Job drawing, mm, ordinate dimensions from the low corner. One solid piece. Coordinates: 2 decimals unless noted, no trailing zeros. Loops run counter-clockwise (first coordinate to the right, second up) from the corner with the lowest first, then second, coordinate; pieces in that order, holes last. Notation, with made-up numbers: (31.5, 59.5) - (39.5, 59.5) arc R26 cw to (39.5, 73.5) - close; hole circle Ø6 at (56, 80.5). An arc over 180 degrees is marked (long way). Use a Markdown table: item, result. Add a question column.
1) Band-saw the part on B-B (x = 5). Give the number of separate pieces and of enclosed holes in the cut face, plus the area to 3 significant figures.
2) Drop flat-ended pins along their axis: P1, Ø6, axis at y = 24, z = 5, coming from the +X side; P2, Ø1, axis at y = 23, z = 7, coming from the -X side; P3, Ø0.8, axis at x = 5, z = 18, coming from the -Y side; P4, Ø7, axis at x = 5, y = 7, coming from the +Z side. Give the stop position or say it passes through.
3) Pull direction Z, two halves, no side cores. Call the marked faces 1, 2 and 3: +Z half, -Z half, draft (parallel to the pull), parting line (faces both ways), or undercut.
4) Band-saw the part on C-C (z = 26). Give the cut face in (x, y), plus the area to 3 significant figures.
5) Band-saw the part on A-A (x = 25.7). Give the cut face in (y, z), plus the area to 3 significant figures.
6) Probe probe 1 along Y at (x, z) = (5, 14.2); probe 2 along Z at (x, y) = (10, 9); probe 3 along Z at (x, y) = (25.7, 15). List the from-to ranges inside material, lowest first. Write a range as [from, to].
7) Band-saw the part on D-D (y = 27). Give the cut face in (x, z), plus the area to 3 significant figures.
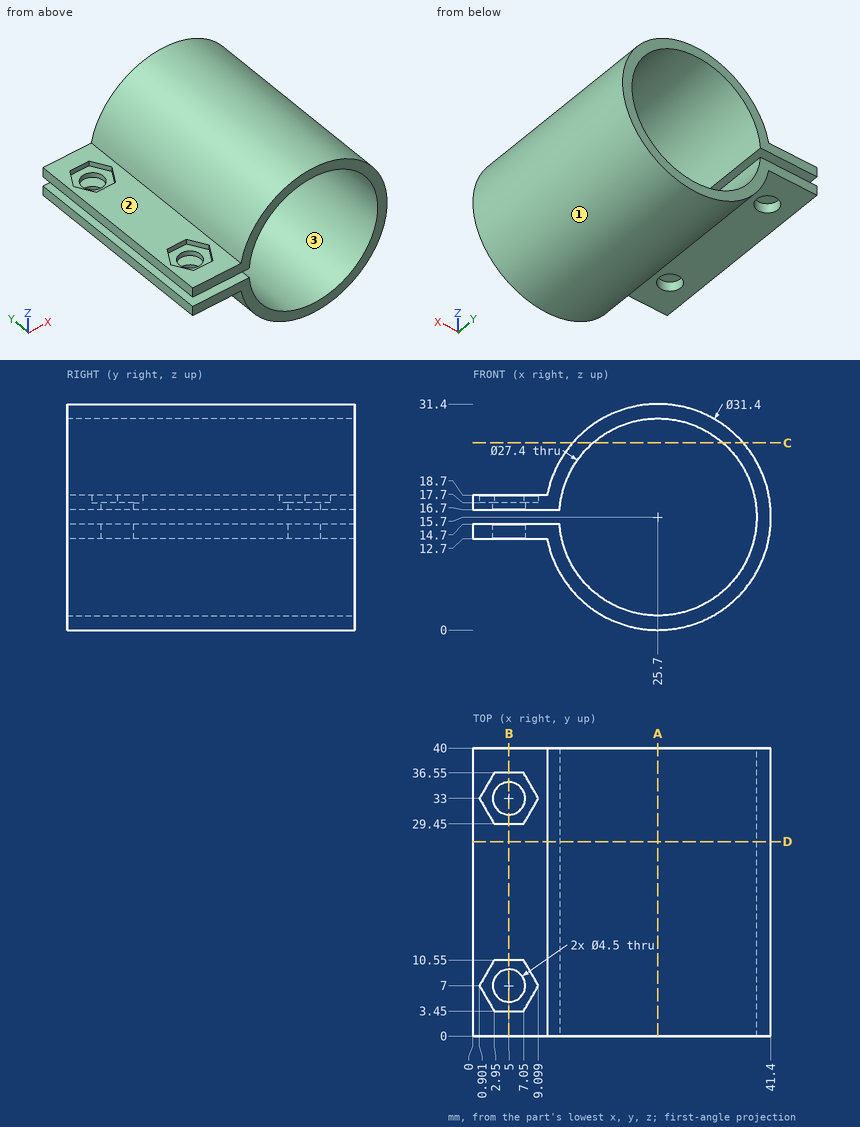
Answer block:
| question | item | result |
|---|---|---|
| 1 | separate pieces | 6 |
| 1 | enclosed holes | 0 |
| 1 | area | 119 mm2 |
| 2 | P1 | x = 39.38 |
| 2 | P2 | x = 12.31 |
| 2 | P3 | y = 0 |
| 2 | P4 | z = 17.7 |
| 3 | face 1 | parting line |
| 3 | face 2 | +Z half |
| 3 | face 3 | undercut |
| 4 | outline | (13.85, 0) - (16.67, 0) - (16.67, 40) - (13.85, 40) - close; (34.73, 0) - (37.55, 0) - (37.55, 40) - (34.73, 40) - close |
| 4 | area | 225 mm2 |
| 5 | outline | (0, 0) - (40, 0) - (40, 2) - (0, 2) - close; (0, 29.4) - (40, 29.4) - (40, 31.4) - (0, 31.4) - close |
| 5 | area | 160 mm2 |
| 6 | probe 1 | [0, 4.75], [9.25, 30.75], [35.25, 40] |
| 6 | probe 2 | [12.7, 14.7], [16.7, 18.7] |
| 6 | probe 3 | [0, 2], [29.4, 31.4] |
| 7 | outline | (0, 12.7) - (10.29, 12.7) arc R15.7 ccw (long way) to (10.29, 18.7) - (0, 18.7) - (0, 16.7) - (12.04, 16.7) arc R13.7 cw (long way) to (12.04, 14.7) - (0, 14.7) - close |
| 7 | area | 221 mm2 |
